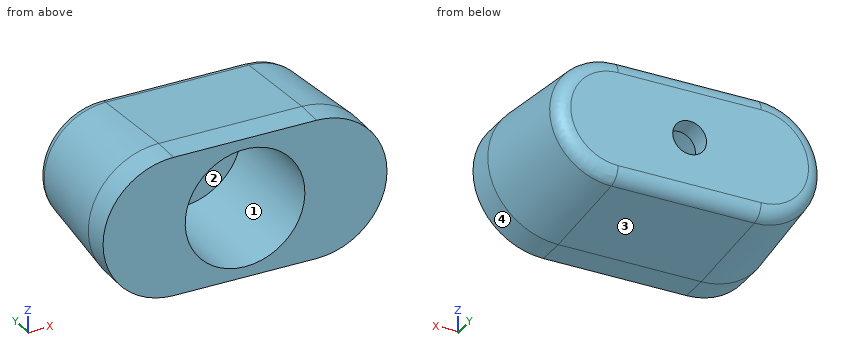
from build123d import *

# Parameters (mm, degrees)
SKETCH1_W           = 102.87
SKETCH1_H           = 52.07
BOSS_EXTRUDE2_DEPTH = 10
BOSS_EXTRUDE3_DEPTH = 40.5
BOSS_EXTRUDE3_TAPER = 5
SKETCH4_R           = 21.25
CUT_EXTRUDE2_DEPTH  = 43
FILLET1_R           = 5.08
SKETCH5_R           = 6
CUT_EXTRUDE3_DEPTH  = 77.639614104
SKETCH6_OUTSIDE_W   = 130.044
SKETCH6_OUTSIDE_H   = 79.244
CUT_EXTRUDE4_DEPTH  = 71.453037195


with BuildPart() as part:
    # Sketch1 → Boss-Extrude2 (new body)
    with BuildSketch(Plane(origin=(0, 0, 0), x_dir=(1, 0, 0), z_dir=(0, 1, 0))):
        Rectangle(SKETCH1_W, SKETCH1_H)
    extrude(amount=BOSS_EXTRUDE2_DEPTH)

    # Sketch3 → Boss-Extrude3 (add)
    with BuildSketch(Plane(origin=(0, 10, 0), x_dir=(1, 0, 0), z_dir=(0, 1, 0))):
        with BuildLine():
            ThreePointArc((-25.4, 25.000000038), (-50.400000038, 0), (-25.4, -25.000000038))
            Line((-25.4, -25.000000038), (25.4, -25.000000038))
            ThreePointArc((25.4, -25.000000038), (50.400000038, 0), (25.4, 25.000000038))
            Line((25.4, 25.000000038), (-25.4, 25.000000038))
        make_face()
    extrude(amount=BOSS_EXTRUDE3_DEPTH, taper=BOSS_EXTRUDE3_TAPER)

    # Sketch4 → Cut-Extrude2 (cut)
    with BuildSketch(Plane.XZ):
        with Locations(Location((0, 0, 0), (0, 0, 270))):
            Circle(SKETCH4_R)
    extrude(amount=-CUT_EXTRUDE2_DEPTH, mode=Mode.SUBTRACT)

    # Fillet1
    fillet1_edges = [part.edges().sort_by_distance(p)[0] for p in [
        (-46.856709165, 50.5, 0),
        (0, 50.5, 21.456709165),
        (46.856709165, 50.5, 0),
        (0, 50.5, -21.456709165),
    ]]
    fillet(fillet1_edges, radius=FILLET1_R)

    # Sketch5 → Cut-Extrude3 (cut, through all)
    with BuildSketch(Plane(origin=(0, 50.5, 0), x_dir=(1, 0, 0), z_dir=(0, 1, 0))):
        with Locations(Location((0, 0, 0), (0, 0, 270))):
            Circle(SKETCH5_R)
    extrude(amount=-CUT_EXTRUDE3_DEPTH, mode=Mode.SUBTRACT)

    # Sketch6 outside → Cut-Extrude4 (cut, through all)
    with BuildSketch(Plane(origin=(0, 10, 0), x_dir=(1, 0, 0), z_dir=(0, 1, 0))):
        Rectangle(SKETCH6_OUTSIDE_W, SKETCH6_OUTSIDE_H)
        with BuildLine():
            Line((-25.4, 25.000000038), (25.4, 25.000000038))
            ThreePointArc((25.4, 25.000000038), (50.400000038, 0), (25.4, -25.000000038))
            Line((25.4, -25.000000038), (-25.4, -25.000000038))
            ThreePointArc((-25.4, -25.000000038), (-50.400000038, 0), (-25.4, 25.000000038))
        make_face(mode=Mode.SUBTRACT)
    extrude(amount=-CUT_EXTRUDE4_DEPTH, mode=Mode.SUBTRACT)


solid = part.part
The model under review builds one solid part; all positions refer to its coordinate system, in mm. Face numbers are marked on the shaded views. Round coordinates to 2 decimals unless told otherwise and drop trailing zeros. Write each loop counter-clockwise with the first axis right and the second up, starting at its lowest first coordinate (ties: lowest second). Pieces come first, ordered by that corner, then holes. Notation, with made-up numbers: (45, -4.75) - (51, -4.75) arc R22 cw to (51, 2.25) - close; hole circle Ø10 at (43, 58). An arc over 180 degrees is marked (long way). One line per item, written item: value. Start each with the question number.
1. Consider section C-C on y = 34. Write out the cut boundary in (x, z), and give its area (3 significant figures).
2. Consider section A-A on x = 0. Write out the cut boundary in (y, z), and give its area (3 significant figures).
3. Consider section B-B on y = 5. Write out the cut boundary in (x, z).
4. The part is to be moulded in two halves that separate along X. For the marked faces 1, 2, 3 and 4, say which applies: released by +X, released by -X, zero draft, split by the parting line, or undercut.
5. To check wall thickness, follow L1, parallel to Y at x = -7.5, z = 5.5; L2, parallel to X at y = 16.5, z = -18; L3, parallel to X at y = 6.5, z = -11. State the ranges of each line that lie inside material, in increasing order. Write a range as from..to.
6. Clearance check with flat-ended pins moving along their axes: P1, Ø1, axis at y = 39.5, z = 19.5, coming from the +X side; P2, Ø11, axis at x = 0, z = 0, coming from the +Y side; P3, Ø5, axis at x = 1.5, z = 12.5, coming from the -Y side; P4, Ø4, axis at y = 16.5, z = -5, coming from the -X side. State where each tip first meets the part, or that it passes through.
Checks:
1. outline: (-25.4, -22.9) - (25.4, -22.9) arc R22.9 ccw to (25.4, 22.9) - (-25.4, 22.9) arc R22.9 ccw to start; hole circle Ø42.5 at (0, 0)
1. area: 2,560 mm^2
2. outline: (0, -25) - (10, -25) - (45.86, -21.86) arc R5.08 ccw to (50.5, -16.8) - (50.5, -6) - (43, -6) - (43, -21.25) - (0, -21.25) - close; (0, 21.25) - (43, 21.25) - (43, 6) - (50.5, 6) - (50.5, 16.8) arc R5.08 ccw to (45.86, 21.86) - (10, 25) - (0, 25) - close
2. area: 455 mm^2
3. outline: (-25.4, -25) - (25.4, -25) arc R25 ccw to (25.4, 25) - (-25.4, 25) arc R25 ccw to start; hole circle Ø42.5 at (0, 0)
4. face 1: undercut
4. face 2: undercut
4. face 3: zero draft
4. face 4: released by +X
5. L1: y = 43..50.5
5. L2: x = -41.92..-11.29, 11.29..41.92
5. L3: x = -47.85..-18.18, 18.18..47.85
6. P1: stops at x = 37.3
6. P2: passes through
6. P3: stops at y = 43
6. P4: stops at x = -49.7
